from build123d import *


with BuildPart() as part:
    # Sketch2 → Revolve1 (revolve)
    with BuildSketch(Plane(origin=(0, 0, 0), x_dir=(1, 0, 0), z_dir=(0, 1, 0)), mode=Mode.PRIVATE) as revolve1_sk:
        Polygon((-99.75, 4.25), (-87.75, 4.25), (-87.75, 5), (42.25, 5), (42.25, 6.5), (44.25, 6.5), (44.25, 5), (87.75, 5), (87.75, 4.25), (99.75, 4.25), (99.75, 0), (-99.75, 0), align=None)
    revolve(revolve1_sk.sketch.rotate(Axis((-69.609903496, 0, 0), (1, 0, 0)), 180), axis=Axis((-69.609903496, 0, 0), (1, 0, 0)))

    # Sketch5 → M4x0.7 Tapped Hole1 (revolve, cut)
    with BuildSketch(Plane(origin=(99.75, 0, 0), x_dir=(0, 0, -1), z_dir=(0, 1, 0))):
        Polygon((0, 0), (0, 15.991420021), (1.65, 15), (1.65, 0), align=None)
    m4x0_7_tapped_hole1 = revolve(axis=Axis((106.1, 0, 0), (-1, 0, 0)), mode=Mode.SUBTRACT)

    # Mirror1: M4x0.7 Tapped Hole1 across plane
    add(m4x0_7_tapped_hole1.mirror(Plane(origin=(0, 0, 0), x_dir=(0, 0, 1), z_dir=(1, 0, 0))), mode=Mode.SUBTRACT)


solid = part.part
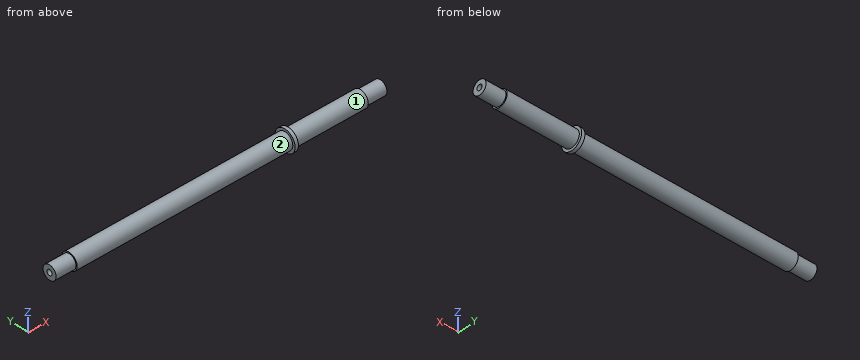
Verification items for the finished model (mm, model axes). Face numbers are marked on the shaded views. A direction names the side the tool comes from. Give positions to 0.01 mm unless a question says otherwise; leave off trailing zeros. Loops run counter-clockwise (first coordinate to the right, second up) from the corner with the lowest first, then second, coordinate; pieces in that order, holes last. Notation, with made-up numbers: (-4.75, 4.5) - (0.25, 4.5) arc R22 ccw to (0.25, 28.5) - close; hole circle Ø9 at (-39, -15.75). An arc over 180 degrees is marked (long way). Write item = value, one per line. Start each with the question number.
Q1. Tool access check on the marked faces 1 and 2. Record the directions out of +Z, -Z, +X, -X, +Y, -Y that give a thin tool (end or side, any length) a straight path to the whole face; none if there is none.
Q2. Depth check by flat-ended pin: P1, Ø1.5, axis at x = 67, z = 1, coming from the -Y side; P2, Ø2, axis at x = -41, y = 2, coming from the -Z side; P3, Ø3, axis at y = 0, z = 0, coming from the -X side. Enter the tip coordinate at first touch or a pass-through.
Q3. Thickness scan on line 1 (Y direction, x = 88.5, z = 0); line 2 (X direction, y = 4.5, z = 0); line 3 (Y direction, x = 85.5, z = 0). Record the ranges inside material, lowest first.
Q4. Cross-section at A-A, the plane x = 65.5. Enter the section's corners in (y, z), and give its area (3 significant figures).
Answer key:
q1.face_1 = +X
q1.face_2 = -X
q2.P1 = -4.99
q2.P2 = -4.9
q2.P3 = -84.66
q3.line_1 = -4.25 to -1.65, 1.65 to 4.25
q3.line_2 = -87.75 to 87.75
q3.line_3 = -5 to -1.65, 1.65 to 5
q4.outline = circle Ø10 at (0, 0)
q4.area = 78.5 mm^2
